Source: three-view drawing plus pictorial views. Frame: mm from the lowest corner of the part. A direction names the side the tool comes from. Give positions to 0.01 mm unless a question says otherwise; leave off trailing zeros. Order: outer loops, then holes, each group sorted by start corner. A loop starts at its lowest first (then second) coordinate and runs counter-clockwise, first axis right, second up. Notation, with made-up numbers: M 1,51.5 L 53,51.5 A15 cw 53,66.5 Z; hole C 20.25,-21 d5. An arc over 180 degrees is marked long. One line per item, written item: value. Start each with the question number.
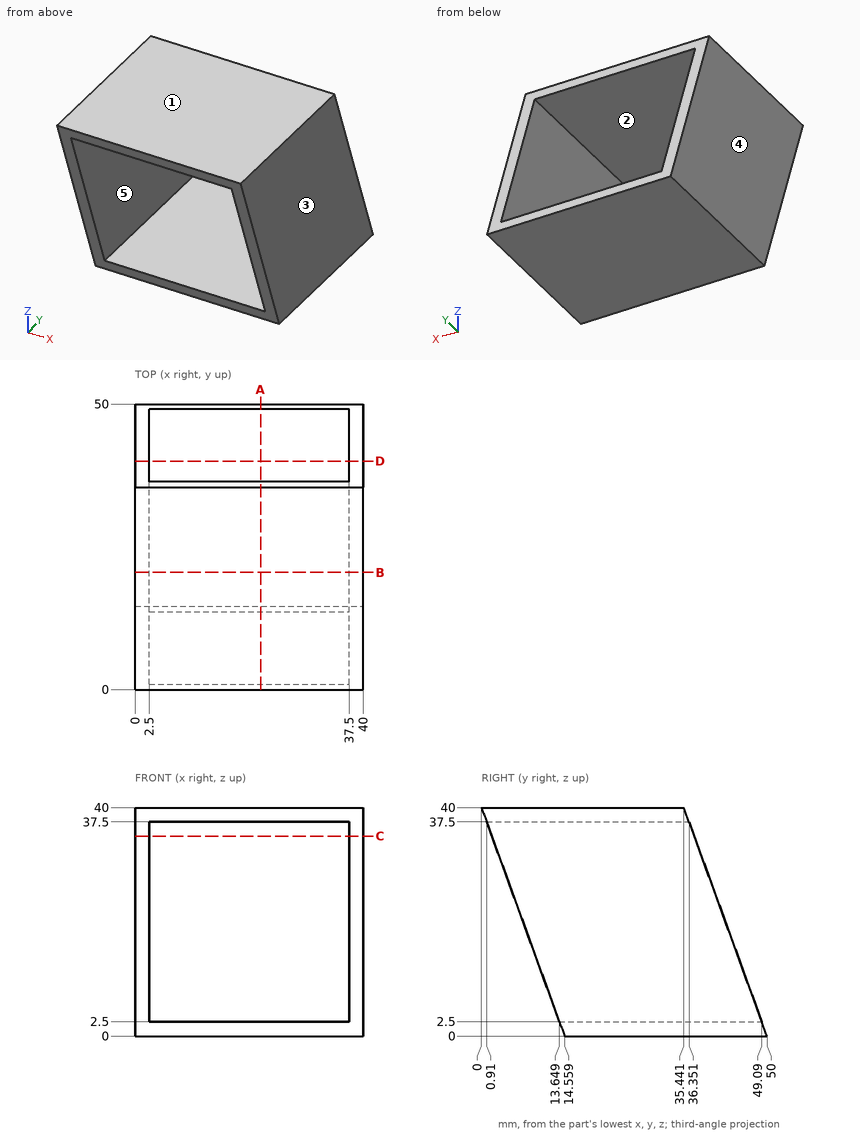
Q1. Contact query for a flat-ended pin moving along its axis: pin 1 (5 mm diameter, centred on x = 33.5, z = 26, fed in from -Y). Output: stop coordinate, or through.
Q2. Mould query, pull axis X, two halves, no side actions, for the marked faces 1, 2 and 3. Classes: +X half, -X half, draft (parallel to the pull), parting line (faces both ways), or undercut.
Q3. Section query C-C on z = 35. Return loops of the section in (x, y).
Q4. Section query B-B on y = 20.5. Return loops of the section in (x, z), and give its area (3 significant figures).
Q5. Set-up query: the marked faces 4 and 5. Return all of +Z, -Z, +X, -X, +Y, -Y with unobstructed straight access to the full face (end or side cutting, diameter ignored); none if empty.
Q6. Section query D-D on y = 40. Return loops of the section in (x, z) (1 decimal).
Q7. Section query A-A on x = 22. Return loops of the section in (y, z).
Q8. Ray query, line 1 along X through (y, z) = (34, 31); line 2 along Z through (x, y) = (9, 9). Return the intervals inside material, ascending. Write a range as [from, to].
Results below:
1. pin 1: through
2. face 1: draft
2. face 2: undercut
2. face 3: +X half
3. outline: M 0,1.82 L 2.5,1.82 L 2.5,37.26 L 0,37.26 Z; M 37.5,1.82 L 40,1.82 L 40,37.26 L 37.5,37.26 Z
4. outline: M 0,0 L 40,0 L 40,40 L 0,40 Z; hole M 2.5,2.5 L 37.5,2.5 L 37.5,37.5 L 2.5,37.5 Z
4. area: 375 mm2
5. face 4: +Z, -Z, -X, +Y, -Y
5. face 5: +Y, -Y
6. outline: M 0,0 L 40,0 L 40,27.5 L 37.5,27.5 L 37.5,2.5 L 2.5,2.5 L 2.5,27.5 L 0,27.5 Z
7. outline: M 0,40 L 0.91,37.5 L 36.35,37.5 L 35.44,40 Z; M 13.65,2.5 L 14.56,0 L 50,0 L 49.09,2.5 Z
8. line 1: [0, 2.5], [37.5, 40]
8. line 2: [37.5, 40]
